Design review of the part built by this model. Coordinates are the model's own, in mm. A direction names the side the tool comes from. Round coordinates to 2 decimals unless told otherwise and drop trailing zeros. Loops run counter-clockwise (first coordinate to the right, second up) from the corner with the lowest first, then second, coordinate; pieces in that order, holes last. Notation, with made-up numbers: M 68.5,10 L 93.5,10 A21 ccw 93.5,23 Z; hole C 77.5,-26 d6. An arc over 180 degrees is marked long. One line per item, written item: value. Start each with the question number.
Item 1: We need section B-B (x = 123). Write out the cut boundary in (y, z), then the cut area to 3 significant figures.
Item 2: For line 1 along Z through (x, y) = (133.5, 9.5); line 2 along X through (y, z) = (9, 86); line 3 along Y through (x, z) = (161.4, 49.53), list the stretches that pass through material, from the lowest coordinate up.
Item 3: For faces 1 (the cylindrical face through (-1.29, 21.52, 76.3)), 2 (the flat face through (113, 5, 17)), 3 (the flat face through (148, 30.798, 70)), list the 3-axis set-ups (+Z, -Z, +X, -X, +Y, -Y) from which the entire face can be reached by the end or side of a thin tool; tool diameter is ignored.
Item 4: Clearance check with flat-ended pins moving along their axes: pin 1 (1.5 mm diameter, centred on y = 33.5, z = 30.5, fed in from +X); pin 2 (2 mm diameter, centred on x = 79.5, y = 29, fed in from -Z); pin 3 (5 mm diameter, centred on x = 114, z = 67, fed in from +Y). State where each tip first meets the part, or that it passes through.
Item 5: We need section A-A (z = 8.89). Write out the cut boundary in (x, y), then the cut area to 3 significant figures.
Item 6: We need section C-C (z = 49.53). Write out the cut boundary in (x, y).
Item 7: We need section D-D (y = 44). Write out the cut boundary in (x, z).
Item 8: Mouldability with a two-part tool opening along Z and no side actions: class faces 4 (the flat face through (148, 30.798, 20)), 5 (the cylindrical face through (-1.29, 16.08, 7.24)) as released by +Z, released by -Z, zero draft, split by the parting line, or undercut.
from build123d import *

# Parameters (mm, degrees)
BOSS_EXTRUDE1_DEPTH  = 2.54
SKETCH2_W            = 152.4
SKETCH2_H            = 93.98
BOSS_EXTRUDE2_DEPTH  = 2.54
BOSS_EXTRUDE3_DEPTH  = 2.54
SKETCH4_W            = 152.4
SKETCH4_H            = 2.54
BOSS_EXTRUDE4_DEPTH  = 2.54
BOSS_EXTRUDE13_DEPTH = 2.54
BOSS_EXTRUDE14_DEPTH = 2.54
SKETCH19_W           = 7.62
SKETCH19_H           = 33.3375
BOSS_EXTRUDE15_DEPTH = 2.54
SKETCH20_W           = 7.62
SKETCH20_H           = 33.3375
BOSS_EXTRUDE16_DEPTH = 2.54
SKETCH21_W           = 93.98
SKETCH21_H           = 2.54
BOSS_EXTRUDE17_DEPTH = 7.62
SKETCH22_W           = 2.54
SKETCH22_H           = 33.3375
BOSS_EXTRUDE18_DEPTH = 99.06
SKETCH23_W           = 99.06
SKETCH23_H           = 49.8475
BOSS_EXTRUDE19_DEPTH = 2.54
SKETCH24_R           = 3.639281935
SKETCH24_R_2         = 7.62
SKETCH24_R_3         = 3.285560526
CUT_EXTRUDE2_DEPTH   = 2.54
SKETCH25_R           = 6.906854853
CUT_EXTRUDE3_DEPTH   = 2.54
SKETCH29_R           = 2
BOSS_EXTRUDE20_DEPTH = 30.7975
SKETCH31_R           = 5
BOSS_EXTRUDE21_DEPTH = 5


with BuildPart() as part:
    # Sketch1 → Boss-Extrude1 (new body)
    with BuildSketch(Plane.XY):
        Polygon((0, 0), (152.4, 0), (152.4, 26.9875), (76.2, 26.9875), (63.5, 43.4975), (0, 43.4975), align=None)
    extrude(amount=BOSS_EXTRUDE1_DEPTH)



with BuildPart() as body_2:
    # Sketch2 → Boss-Extrude2 (new body)
    with BuildSketch(Plane(origin=(0, 0, 0), x_dir=(-1, 0, 0), z_dir=(0, -1, 0))):
        with Locations((-76.2, -49.53)):
            Rectangle(SKETCH2_W, SKETCH2_H)
    extrude(amount=BOSS_EXTRUDE2_DEPTH)

    # Sketch3 → Boss-Extrude3 (add)
    with BuildSketch(Plane.XY.offset(96.52)):
        Polygon((0, 0), (0, 43.4975), (63.5, 43.4975), (76.2, 26.9875), (152.4, 26.9875), (152.4, -2.54), (0, -2.54), align=None)
    extrude(amount=BOSS_EXTRUDE3_DEPTH)


with BuildPart() as part_1:
    add(part.part)

    add(body_2.part)  # Boss-Extrude4 merges body 2
    # Sketch4 → Boss-Extrude4 (add)
    with BuildSketch(Plane(origin=(0, 0, 2.54), x_dir=(-1, 0, 0), z_dir=(0, 0, -1))):
        with Locations((-76.2, -1.27)):
            Rectangle(SKETCH4_W, SKETCH4_H)
    extrude(amount=BOSS_EXTRUDE4_DEPTH)

    # Sketch10 → Boss-Extrude13 (add)
    with BuildSketch(Plane(origin=(0, 0, 0), x_dir=(-1, 0, 0), z_dir=(0, 0, -1))):
        Polygon((0, 43.4975), (0, 47.3075), (-63.5, 47.3075), (-76.2, 30.7975), (-152.4, 30.7975), (-152.4, 26.9875), (-76.2, 26.9875), (-63.5, 43.4975), align=None)
    extrude(amount=-BOSS_EXTRUDE13_DEPTH)

    # Sketch18 → Boss-Extrude14 (add)
    with BuildSketch(Plane.XY.offset(99.06)):
        Polygon((0, 43.4975), (0, 47.3075), (63.5, 47.3075), (76.2, 30.7975), (152.4, 30.7975), (152.4, 26.9875), (76.2, 26.9875), (63.5, 43.4975), align=None)
    extrude(amount=-BOSS_EXTRUDE14_DEPTH)

    # Sketch19 → Boss-Extrude15 (add)
    with BuildSketch(Plane.XY.offset(99.06)):
        with Locations((156.21, 14.12875)):
            Rectangle(SKETCH19_W, SKETCH19_H)
    extrude(amount=-BOSS_EXTRUDE15_DEPTH)

    # Sketch20 → Boss-Extrude16 (add)
    with BuildSketch(Plane(origin=(0, 0, 0), x_dir=(-1, 0, 0), z_dir=(0, 0, -1))):
        with Locations((-156.21, 14.12875)):
            Rectangle(SKETCH20_W, SKETCH20_H)
    extrude(amount=-BOSS_EXTRUDE16_DEPTH)

    # Sketch21 → Boss-Extrude17 (add)
    with BuildSketch(Plane(origin=(152.4, 0, 0), x_dir=(0, 0, -1), z_dir=(1, 0, 0))):
        with Locations((-49.53, -1.27)):
            Rectangle(SKETCH21_W, SKETCH21_H)
    extrude(amount=BOSS_EXTRUDE17_DEPTH)

    # Sketch22 → Boss-Extrude18 (add)
    with BuildSketch(Plane.XY.offset(99.06)):
        with Locations((161.29, 14.12875)):
            Rectangle(SKETCH22_W, SKETCH22_H)
    extrude(amount=-BOSS_EXTRUDE18_DEPTH)

    # Sketch23 → Boss-Extrude19 (add)
    with BuildSketch(Plane.ZY):
        with Locations((49.53, 22.38375)):
            Rectangle(SKETCH23_W, SKETCH23_H)
    extrude(amount=BOSS_EXTRUDE19_DEPTH)

    # Sketch24 → Cut-Extrude2 (cut)
    with BuildSketch(Plane.ZY.offset(2.54)):
        with Locations((58.358660758, 23.518484008)):
            Circle(SKETCH24_R)
        with Locations((8.89, 23.518484008)):
            Circle(SKETCH24_R_2)
        with Locations((78.906077051, 23.518484008)):
            Circle(SKETCH24_R_3)
    extrude(amount=-CUT_EXTRUDE2_DEPTH, mode=Mode.SUBTRACT)

    # Sketch25 → Cut-Extrude3 (cut)
    with BuildSketch(Plane(origin=(162.56, 0, 0), x_dir=(0, 0, -1), z_dir=(1, 0, 0))):
        with Locations((-49.53, 14.12875)):
            Circle(SKETCH25_R)
    extrude(amount=-CUT_EXTRUDE3_DEPTH, mode=Mode.SUBTRACT)

    # Sketch29 → Boss-Extrude20 (add)
    with BuildSketch(Plane(origin=(0, 0, 0), x_dir=(1, 0, 0), z_dir=(0, 1, 0))):
        with Locations(Location((112.968, -19.540242478, 0), (0, 0, 90))):
            Circle(SKETCH29_R)
        with Locations(Location((148.02, -19.540242478, 0), (0, 0, 90))):
            Circle(SKETCH29_R)
        with Locations(Location((112.968, -69.578242478, 0), (0, 0, 90))):
            Circle(SKETCH29_R)
        with Locations(Location((148.02, -69.578242478, 0), (0, 0, 90))):
            Circle(SKETCH29_R)
    extrude(amount=BOSS_EXTRUDE20_DEPTH)

    # Sketch31 → Boss-Extrude21 (add)
    with BuildSketch(Plane(origin=(0, 0, 0), x_dir=(1, 0, 0), z_dir=(0, 1, 0))):
        with Locations(Location((112.968, -19.540242478, 0), (0, 0, 90))):
            Circle(SKETCH31_R)
        with Locations(Location((148.02, -19.540242478, 0), (0, 0, 90))):
            Circle(SKETCH31_R)
        with Locations(Location((112.968, -69.578242478, 0), (0, 0, 90))):
            Circle(SKETCH31_R)
        with Locations(Location((148.02, -69.578242478, 0), (0, 0, 90))):
            Circle(SKETCH31_R)
    extrude(amount=BOSS_EXTRUDE21_DEPTH)


solid = part_1.part
A:
1. outline: M -2.54,0 L 30.8,0 L 30.8,2.54 L 0,2.54 L 0,96.52 L 30.8,96.52 L 30.8,99.06 L -2.54,99.06 Z
1. area: 408 mm2
2. line 1: 0 to 2.54, 96.52 to 99.06
2. line 2: -2.54 to 0, 160.02 to 162.56
2. line 3: -2.54 to 7.22, 21.04 to 30.8
3. face 1: -X
3. face 2: +Y
3. face 3: +Z, -Z, +X, +Y
4. pin 1: x = 0
4. pin 2: z = 0
4. pin 3: y = 30.8
5. outline: M -2.54,-2.54 L 162.56,-2.54 L 162.56,30.8 L 160.02,30.8 L 160.02,0 L 0,0 L 0,15.9 L -2.54,15.9 Z; M -2.54,31.14 L 0,31.14 L 0,47.31 L -2.54,47.31 Z
5. area: 579 mm2
6. outline: M -2.54,-2.54 L 162.56,-2.54 L 162.56,7.22 L 160.02,7.22 L 160.02,0 L 0,0 L 0,47.31 L -2.54,47.31 Z; M 160.02,21.04 L 162.56,21.04 L 162.56,30.8 L 160.02,30.8 Z
7. outline: M -2.54,0 L 66.04,0 L 66.04,2.54 L 0,2.54 L 0,96.52 L 66.04,96.52 L 66.04,99.06 L -2.54,99.06 Z
8. face 4: zero draft
8. face 5: undercut
